Geometry check sheet. Reference: the model listing, model coordinates, mm. A direction names the side the tool comes from. Round coordinates to 2 decimals unless told otherwise and drop trailing zeros. Write each loop counter-clockwise with the first axis right and the second up, starting at its lowest first coordinate (ties: lowest second). Pieces come first, ordered by that corner, then holes. Notation, with made-up numbers: (84, -2.75) -> (105, -2.75) arc R20 ccw to (105, 7.25) -> close; hole circle Ø7 at (-28, -9). An arc over 180 degrees is marked (long way). Use a Markdown table: item, result.
```python
from build123d import *

# Parameters (mm, degrees)
F_3MM_DEPTH           = 3
CUT_EXTRUDE_368_DEPTH = 3
D6P4_1_7_2_START      = 7.2
SKETCH_3_R            = 5.5
SKETCH_3_R_2          = 3.2
D6P4_1_7_2_DEPTH      = 9.8
D6P4_1_67_START       = 67
SKETCH_4_R            = 5.5
SKETCH_4_R_2          = 3.2
D6P4_1_67_DEPTH       = 9.8
SKETCH_5_R            = 5.5
SKETCH_5_R_2          = 3.2
D6P4_1_7_2_2_DEPTH    = 9.8
SKETCH_6_R            = 5.5
SKETCH_6_R_2          = 3.2
D6P4_1_67_2_DEPTH     = 9.8


with BuildPart() as part:
    # 草图1 → 斜切侧罩_3mm外壳 (new body)
    with BuildSketch(Plane.XY):
        Polygon((-62, 7.5), (62, 7.5), (68, 13.5), (68, 70.5), (62, 76.5), (-62, 76.5), (-68, 70.5), (-68, 13.5), align=None)
    extrude(amount=F_3MM_DEPTH)

    # 草图2 → Cut-Extrude 368 (cut)
    with BuildSketch(Plane.XY):
        Polygon((-58, 11.5), (58, 11.5), (60, 13.5), (60, 35), (56, 39), (-56, 39), (-60, 35), (-60, 13.5), align=None)
        Polygon((-22, 43), (22, 43), (58, 77.5), (-58, 77.5), align=None)
        Polygon((-30, 43), (-60, 43), (-60, 69), align=None)
        Polygon((30, 43), (60, 43), (60, 69), align=None)
    extrude(amount=CUT_EXTRUDE_368_DEPTH, mode=Mode.SUBTRACT)

    # 草图3 → D6p4_-1_7.2 (add)
    with BuildSketch(Plane(origin=(0, 0, 0), x_dir=(1, 0, 0), z_dir=(0, 1, 0)).offset(D6P4_1_7_2_START)):
        with Locations(Location((-62, 4, 0), (0, 0, 270))):
            Circle(SKETCH_3_R)
        with Locations(Location((-62, 4, 0), (0, 0, 270))):
            Circle(SKETCH_3_R_2, mode=Mode.SUBTRACT)
    extrude(amount=D6P4_1_7_2_DEPTH)

    # 草图4 → D6p4_-1_67 (add)
    with BuildSketch(Plane(origin=(0, 0, 0), x_dir=(1, 0, 0), z_dir=(0, 1, 0)).offset(D6P4_1_67_START)):
        with Locations(Location((-62, 4, 0), (0, 0, 270))):
            Circle(SKETCH_4_R)
        with Locations(Location((-62, 4, 0), (0, 0, 270))):
            Circle(SKETCH_4_R_2, mode=Mode.SUBTRACT)
    extrude(amount=D6P4_1_67_DEPTH)

    # 草图5 → D6p4_1_7.2 2 (add)
    with BuildSketch(Plane(origin=(0, 0, 0), x_dir=(1, 0, 0), z_dir=(0, 1, 0)).offset(D6P4_1_7_2_START)):
        with Locations(Location((62, 4, 0), (0, 0, 270))):
            Circle(SKETCH_5_R)
        with Locations(Location((62, 4, 0), (0, 0, 270))):
            Circle(SKETCH_5_R_2, mode=Mode.SUBTRACT)
    extrude(amount=D6P4_1_7_2_2_DEPTH)

    # 草图6 → D6p4_1_67 2 (add)
    with BuildSketch(Plane(origin=(0, 0, 0), x_dir=(1, 0, 0), z_dir=(0, 1, 0)).offset(D6P4_1_67_START)):
        with Locations(Location((62, 4, 0), (0, 0, 270))):
            Circle(SKETCH_6_R)
        with Locations(Location((62, 4, 0), (0, 0, 270))):
            Circle(SKETCH_6_R_2, mode=Mode.SUBTRACT)
    extrude(amount=D6P4_1_67_2_DEPTH)


solid = part.part
```
(1) Section check A-A on x = 35.5. Record the cut outline in (y, z).
A:
| item | result |
|---|---|
| outline | (7.5, 0) -> (11.5, 0) -> (11.5, 3) -> (7.5, 3) -> close; (39, 0) -> (43, 0) -> (43, 3) -> (39, 3) -> close; (47.77, 0) -> (55.94, 0) -> (55.94, 3) -> (47.77, 3) -> close |
(2) Section check B-B on x = 3.5. Record the cut outline in (y, z).
A:
| item | result |
|---|---|
| outline | (7.5, 0) -> (11.5, 0) -> (11.5, 3) -> (7.5, 3) -> close; (39, 0) -> (43, 0) -> (43, 3) -> (39, 3) -> close |
(3) Section check D-D on x = -32. Record the cut outline in (y, z).
A:
| item | result |
|---|---|
| outline | (7.5, 0) -> (11.5, 0) -> (11.5, 3) -> (7.5, 3) -> close; (39, 0) -> (43, 0) -> (43, 3) -> (39, 3) -> close; (44.73, 0) -> (52.58, 0) -> (52.58, 3) -> (44.73, 3) -> close |
(4) Access from +Z, -Z, +X, -X, +Y, -Y to the whole of each face (thin tool, end or side, straight path). Record for faces 1 (the face through (58, 37, 1)), 2 (the face through (59.6, 7.2, -1.6)).
A:
| item | result |
|---|---|
| face 1 | +Z, -Z |
| face 2 | +Z, -Z, +X, -X, -Y |
(5) Thickness scan on line 1 (X direction, y = 9.75, z = -4); line 2 (X direction, y = 21.5, z = 2); line 3 (Y direction, x = 42.5, z = 2.75). Record the ranges inside material, lowest first.
A:
| item | result |
|---|---|
| line 1 | x = -67.5 to -65.2, -58.8 to -56.5, 56.5 to 58.8, 65.2 to 67.5 |
| line 2 | x = -68 to -60, 60 to 68 |
| line 3 | y = 7.5 to 11.5, 39 to 43, 53.83 to 62.65 |
(6) Gauge pin test, flat ends, axial feed: pin 1 Ø0.9 at (x, z) = (-18, 2) entering from +Y; pin 2 Ø3.5 at (x, z) = (-44, 1.5) entering from +Y; pin 3 Ø1.5 at (x, z) = (22, 2) entering from -Y. Record the tip position at first contact, or that the pin passes through.
A:
| item | result |
|---|---|
| pin 1 | stops at y = 43 |
| pin 2 | stops at y = 65.76 |
| pin 3 | stops at y = 7.5 |
(7) Section check C-C on y = 64.5. Record the cut outline in (x, z).
A:
| item | result |
|---|---|
| outline | (-68, 0) -> (-60, 0) -> (-60, 3) -> (-68, 3) -> close; (-54.81, 0) -> (-44.43, 0) -> (-44.43, 3) -> (-54.81, 3) -> close; (44.43, 0) -> (54.81, 0) -> (54.81, 3) -> (44.43, 3) -> close; (60, 0) -> (68, 0) -> (68, 3) -> (60, 3) -> close |
(8) Release check for a two-part mould opening along X. For faces 3 (the face through (-64.839, 71.831, -2.523)), 4 (the face through (-65.6, 72.9, 1.8)), 5 (the face through (0, 40, 3)) record: +X half, -X half, draft (parallel to the pull), parting line (faces both ways), or undercut.
A:
| item | result |
|---|---|
| face 3 | undercut |
| face 4 | -X half |
| face 5 | draft |
